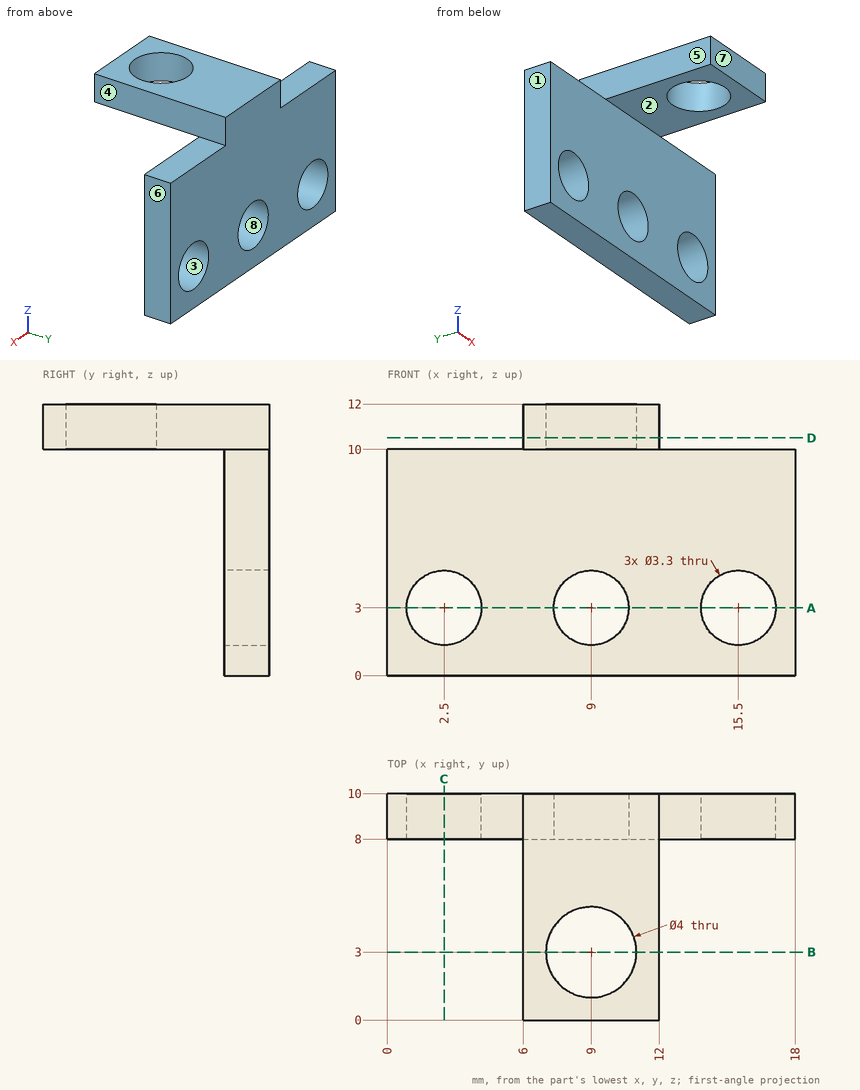
Study the drawing (mm; zero at the part's minimum x, y, z) and answer. A direction names the side the tool comes from. Round coordinates to 2 decimals unless told otherwise and drop trailing zeros. Write each loop counter-clockwise with the first axis right and the second up, starting at its lowest first coordinate (ties: lowest second). Pieces come first, ordered by that corner, then holes. Notation, with made-up numbers: (49, 39.5) -> (88, 39.5) arc R19 ccw to (88, 58.5) -> close; hole circle Ø7 at (-8, 7). An arc over 180 degrees is marked (long way). Answer as CSV lines item,"result". Start each with the question number.
(1) The part is cut by section A-A, the plane z = 3. Give the vertices of the cut face in (x, y), then the cut area to 3 significant figures.
(2) The part is cut by section C-C, the plane x = 2.5. Give the vertices of the cut face in (y, z), then the cut area to 3 significant figures.
(3) A tool of negligible diameter and unlimited length cuts with its end or side. For the marked faces 1, 2, 3, 4 and 5, from which of +Z, -Z, +X, -X, +Y, -Y can it reach the whole face along a straight path? Write none if from no direction.
(4) Find the intervals of material crossed by probe 1 along X at (y, z) = (9.15, 3); probe 2 along Y at (x, z) = (9, 11.6); probe 3 along Y at (x, z) = (11.75, 3.25), in increasing order.
(5) The part is cut by section D-D, the plane z = 10.5. Give the vertices of the cut face in (x, y), then the cut area to 3 significant figures.
(6) The part is cut by section B-B, the plane y = 3. Give the vertices of the cut face in (x, z), then the cut area to 3 significant figures.
(7) The mould has two halves that part along X. Classify the marked faces 6, 7 and 8: +X half, -X half, draft (parallel to the pull), parting line (faces both ways), or undercut.
(8) Each of these flat-tipped pins is pushed along its axis until it touches: pin 1 (3 mm diameter, centred on y = 5, z = 10.5, fed in from -X); pin 2 (0.6 mm diameter, centred on x = 3, y = 9.5, fed in from +Z); pin 3 (1 mm diameter, centred on x = 14, z = 9, fed in from -Y). Where does it stop, or does it pass through?
Output values:
1,outline,"(0, 8) -> (0.85, 8) -> (0.85, 10) -> (0, 10) -> close; (4.15, 8) -> (7.35, 8) -> (7.35, 10) -> (4.15, 10) -> close; (10.65, 8) -> (13.85, 8) -> (13.85, 10) -> (10.65, 10) -> close; (17.15, 8) -> (18, 8) -> (18, 10) -> (17.15, 10) -> close"
1,area,"16.2 mm²"
2,outline,"(8, 0) -> (10, 0) -> (10, 1.35) -> (8, 1.35) -> close; (8, 4.65) -> (10, 4.65) -> (10, 10) -> (8, 10) -> close"
2,area,"13.4 mm²"
3,face 1,"+Z, -Z, -X, +Y, -Y"
3,face 2,"-Z, +X, -X, -Y"
3,face 3,"+Y, -Y"
3,face 4,"+Z, +X, +Y, -Y"
3,face 5,"+Z, -X, +Y, -Y"
4,probe 1,"x = 0 to 0.85, 4.15 to 7.35, 10.65 to 13.85, 17.15 to 18"
4,probe 2,"y = 0 to 1, 5 to 10"
4,probe 3,"y = 8 to 10"
5,outline,"(6, 0) -> (12, 0) -> (12, 10) -> (6, 10) -> close; hole circle Ø4 at (9, 3)"
5,area,"47.4 mm²"
6,outline,"(6, 10) -> (7, 10) -> (7, 12) -> (6, 12) -> close; (11, 10) -> (12, 10) -> (12, 12) -> (11, 12) -> close"
6,area,"4.00 mm²"
7,face 6,"+X half"
7,face 7,"draft"
7,face 8,"undercut"
8,pin 1,"stops at x = 6"
8,pin 2,"stops at z = 10"
8,pin 3,"stops at y = 8"
